Drawing for the job (mm, zero at the part's lowest x, y, z). A direction names the side the tool comes from. Round coordinates to 2 decimals unless told otherwise and drop trailing zeros. Write each loop counter-clockwise with the first axis right and the second up, starting at its lowest first coordinate (ties: lowest second). Pieces come first, ordered by that corner, then holes.
Item 1: Drop flat-ended pins along their axis: pin 1 Ø1 at (x, y) = (2.5, 0.5) entering from -Z; pin 2 Ø1.6 at (y, z) = (1, 9) entering from -X; pin 3 Ø1.6 at (x, y) = (4.5, 2) entering from +Z. Give the stop position or say it passes through.
Item 2: Mould opens along Z. For the marked faces 4, 5 and 6 say: +Z half, -Z half, draft (parallel to the pull), parting line (faces both ways), or undercut.
Item 3: 3-axis set-ups, long thin cutter, end or side, ignore diameter. For the marked faces 1, 2 and 3: which of +Z, -Z, +X, -X, +Y, -Y reach the whole face in a straight line?
Item 4: Wall check: probe 1 along Z at (x, y) = (5.5, 1.75) (1 decimal); probe 2 along Y at (x, z) = (9, 2.5) (1 decimal); probe 3 along X at (y, z) = (0.9, 3.25). Give the ranges that are in metal, low to high.
Item 5: Band-saw the part on B-B, the plane x = 3.75. Write the cut outline in (y, z) (1 decimal).
Item 6: Band-saw the part on D-D, the plane y = 2.6. Count the separate pieces of the cut face and the enclosed holes in it.
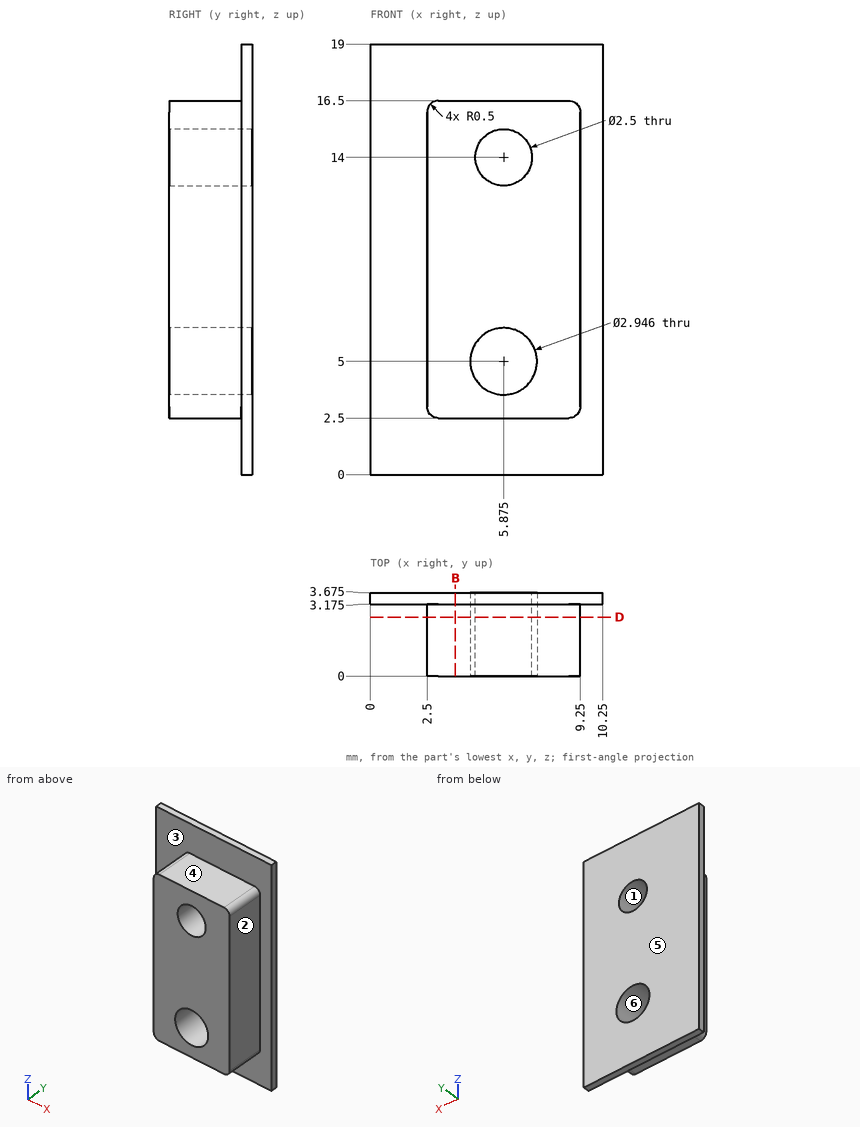
Results:
1. pin 1: stops at z = 2.5
1. pin 2: stops at x = 2.5
1. pin 3: stops at z = 16.5
2. face 4: +Z half
2. face 5: draft
2. face 6: undercut
3. face 1: +Y, -Y
3. face 2: +Z, -Z, +X, -Y
3. face 3: -Y
4. probe 1: z = 2.5 to 3.6, 6.4 to 12.8, 15.2 to 16.5
4. probe 2: y = 3.2 to 3.7
4. probe 3: x = 2.5 to 9.25
5. outline: (0, 2.5) - (3.2, 2.5) - (3.2, 0) - (3.7, 0) - (3.7, 19) - (3.2, 19) - (3.2, 16.5) - (0, 16.5) - close
6. separate pieces: 1
6. enclosed holes: 2
